Autodesk Inventor part; units mm, degrees
ref_plane "a1_XY" through (0, 12.7, -25.2476) normal (0, 1, 0) x (1, 0, 0)
ref_plane "a1_YZ" through (0, 12.7, -25.2476) normal (1, 0, 0) x (0, 0, -1)
ref_plane "a1_ZX" through (0, 12.7, -25.2476) normal (0, 0, -1) x (0, 1, 0)
sketch "Sketch_1" plane through (0, 0, 0) normal (0, 0, 1) x (1, 0, 0)
  line L0 (0, 0) -> (0, 12.7)
  line L1 (0, 12.7) -> (25.2476, 12.7)
  line L2 (25.2476, 12.7) -> (25.2476, 0)
  line L3 (25.2476, 0) -> (0, 0)
  line L4 (0, 0) -> (0, 12.7)
revolve "Revolution1" add sketch "Sketch_1" angle 360 about axis through (0, 0, 0) along (0, -1, 0)
sketch "Sketch_84" plane through (0, 0, 0) normal (0, 0, 1) x (1, 0, 0)
  line L0 (-16.2306, 5.588) -> (-25.2476, 5.588)
  line L1 (-25.2476, 5.588) -> (-25.2476, 11.0427)
  line L2 (-25.2476, 11.0427) -> (-24.6126, 10.4077)
  line L3 (-24.6126, 10.4077) -> (-16.2306, 10.146)
  line L4 (-16.2306, 10.146) -> (-16.2306, 5.588)
  line L5 (-16.2306, 5.588) -> (-25.2476, 5.588)
revolve "Revolution2" cut sketch "Sketch_84" angle 360 about axis through (-16.2306, 5.588, 0) along (1, 0, 0)
thread "Thread1"
sketch "Sketch_85" plane through (0, 0, 0) normal (0, 0, 1) x (1, 0, 0)
  line L0 (-12.2936, 8.8138) -> (-25.2476, 8.8138)
  line L1 (-25.2476, 8.8138) -> (-25.2476, 10.4013)
  line L2 (-25.2476, 10.4013) -> (-13.2101, 10.4013)
  line L3 (-13.2101, 10.4013) -> (-12.2936, 8.8138)
  line L4 (-12.2936, 8.8138) -> (-25.2476, 8.8138)
revolve "Revolution3" cut sketch "Sketch_85" angle 360 about axis through (-12.2936, 8.8138, 0) along (1, 0, 0)
sketch "Sketch4" plane through (0, 12.7, 0) normal (0, 1, 0) x (1, 0, 0)
  point P0 (-15.1587, -15.1587)
hole "Hole1" at (-15.1587, 12.7, 15.1587) direction (0, -1, 0) diameter 3.9624 depth 12.7 counterbore diameter 5.7404 counterbore depth 3.7592
sketch "Sketch5" plane through (0, 12.7, 0) normal (0, 1, 0) x (1, 0, 0)
  point P0 (15.1587, -15.1587)
hole "Hole2" at (15.1587, 12.7, 15.1587) direction (0, -1, 0) diameter 3.9624 depth 12.7 counterbore diameter 5.7404 counterbore depth 3.7592
sketch "Sketch6" plane through (0, 12.7, 0) normal (0, 1, 0) x (1, 0, 0)
  point P0 (15.1587, 15.1587)
hole "Hole3" at (15.1587, 12.7, -15.1587) direction (0, -1, 0) diameter 3.9624 depth 12.7 counterbore diameter 5.7404 counterbore depth 3.7592
sketch "Sketch7" plane through (0, 12.7, 0) normal (0, 1, 0) x (1, 0, 0)
  point P0 (-15.1587, 15.1587)
hole "Hole4" at (-15.1587, 12.7, -15.1587) direction (0, -1, 0) diameter 3.9624 depth 12.7 counterbore diameter 5.7404 counterbore depth 3.7592
sketch "Sketch8" plane through (0, 0, 0) normal (0, -1, 0) x (1, 0, 0)
  point P0 (0, 0)
hole "Hole5" at (0, 0, 0) direction (0, 1, 0) diameter 28.4988 depth 5.5372
sketch "Sketch9" plane through (0, 12.7, 0) normal (0, 1, 0) x (1, 0, 0)
  point P0 (-18.257, -7.5623)
hole "Hole6" at (-18.257, 12.7, 7.5623) direction (0, -1, 0) diameter 2.6416 depth 12.7 counterbore diameter 3.81 counterbore depth 2.54
pattern_linear "Rectangular Pattern1" count 2 spacing 27.9466 along (0.3827, 0, -0.9239) count 2 spacing 27.9466 along (0.9239, 0, 0.3827) of "Hole6"
ref_plane "a1_XY" through (0, 12.7, -25.2476) normal (0, 1, 0) x (1, 0, 0)
ref_plane "a1_YZ" through (0, 12.7, -25.2476) normal (1, 0, 0) x (0, 0, -1)
ref_plane "a1_ZX" through (0, 12.7, -25.2476) normal (0, 0, -1) x (0, 1, 0)
ref_plane "a2_XY" through (0, 12.7, 25.2476) normal (0, 1, 0) x (1, 0, 0)
ref_plane "a2_YZ" through (0, 12.7, 25.2476) normal (1, 0, 0) x (0, 0, -1)
ref_plane "a2_ZX" through (0, 12.7, 25.2476) normal (0, 0, -1) x (0, 1, 0)
ref_plane "ar3_XY" through (-19.8292, 5.5372, 8.2135) normal (0, 1, 0) x (1, 0, 0)
ref_plane "ar3_YZ" through (-19.8292, 5.5372, 8.2135) normal (1, 0, 0) x (0, 0, -1)
ref_plane "ar3_ZX" through (-19.8292, 5.5372, 8.2135) normal (0, 0, -1) x (0, 1, 0)
ref_plane "ar4_XY" through (8.2135, 5.5372, 19.8292) normal (0, 1, 0) x (1, 0, 0)
ref_plane "ar4_YZ" through (8.2135, 5.5372, 19.8292) normal (1, 0, 0) x (0, 0, -1)
ref_plane "ar4_ZX" through (8.2135, 5.5372, 19.8292) normal (0, 0, -1) x (0, 1, 0)
ref_plane "ar5_XY" through (19.8292, 5.5372, -8.2135) normal (0, 1, 0) x (1, 0, 0)
ref_plane "ar5_YZ" through (19.8292, 5.5372, -8.2135) normal (1, 0, 0) x (0, 0, -1)
ref_plane "ar5_ZX" through (19.8292, 5.5372, -8.2135) normal (0, 0, -1) x (0, 1, 0)
ref_plane "ar6_XY" through (-8.2135, 5.5372, -19.8292) normal (0, 1, 0) x (1, 0, 0)
ref_plane "ar6_YZ" through (-8.2135, 5.5372, -19.8292) normal (1, 0, 0) x (0, 0, -1)
ref_plane "ar6_ZX" through (-8.2135, 5.5372, -19.8292) normal (0, 0, -1) x (0, 1, 0)
ref_plane "b1_XY" through (0, 12.7, 0) normal (0, 1, 0) x (1, 0, 0)
ref_plane "b1_YZ" through (0, 12.7, 0) normal (1, 0, 0) x (0, 0, -1)
ref_plane "b1_ZX" through (0, 12.7, 0) normal (0, 0, -1) x (0, 1, 0)
ref_plane "c11_XY" through (15.1587, 12.7, 15.1587) normal (0, 1, 0) x (1, 0, 0)
ref_plane "c11_YZ" through (15.1587, 12.7, 15.1587) normal (1, 0, 0) x (0, 0, -1)
ref_plane "c11_ZX" through (15.1587, 12.7, 15.1587) normal (0, 0, -1) x (0, 1, 0)
ref_plane "c22_XY" through (-15.1587, 12.7, -15.1587) normal (0, 1, 0) x (1, 0, 0)
ref_plane "c22_YZ" through (-15.1587, 12.7, -15.1587) normal (1, 0, 0) x (0, 0, -1)
ref_plane "c22_ZX" through (-15.1587, 12.7, -15.1587) normal (0, 0, -1) x (0, 1, 0)
ref_plane "d11_XY" through (-16.5596, 12.7, -13.7578) normal (0, 1, 0) x (1, 0, 0)
ref_plane "d11_YZ" through (-16.5596, 12.7, -13.7578) normal (1, 0, 0) x (0, 0, -1)
ref_plane "d11_ZX" through (-16.5596, 12.7, -13.7578) normal (0, 0, -1) x (0, 1, 0)
ref_plane "d22_XY" through (-13.7578, 12.7, -16.5596) normal (0, 1, 0) x (1, 0, 0)
ref_plane "d22_YZ" through (-13.7578, 12.7, -16.5596) normal (1, 0, 0) x (0, 0, -1)
ref_plane "d22_ZX" through (-13.7578, 12.7, -16.5596) normal (0, 0, -1) x (0, 1, 0)
ref_plane "j_XY" through (0, 0, 0) normal (0, 1, 0) x (1, 0, 0)
ref_plane "j_YZ" through (0, 0, 0) normal (1, 0, 0) x (0, 0, -1)
ref_plane "j_ZX" through (0, 0, 0) normal (0, 0, -1) x (0, 1, 0)
ref_plane "k1_XY" through (-25.2476, 5.588, 0) normal (0, 0, 1) x (1, 0, 0)
ref_plane "k1_YZ" through (-25.2476, 5.588, 0) normal (1, 0, 0) x (0, 1, 0)
ref_plane "k1_ZX" through (-25.2476, 5.588, 0) normal (0, 1, 0) x (0, 0, 1)
ref_plane "k2_XY" through (-25.2476, 12.7, 0) normal (0, 0, 1) x (1, 0, 0)
ref_plane "k2_YZ" through (-25.2476, 12.7, 0) normal (1, 0, 0) x (0, 1, 0)
ref_plane "k2_ZX" through (-25.2476, 12.7, 0) normal (0, 1, 0) x (0, 0, 1)
ref_plane "po1_XY" through (19.7612, 0, 0) normal (0, 1, 0) x (1, 0, 0)
ref_plane "po1_YZ" through (19.7612, 0, 0) normal (1, 0, 0) x (0, 0, -1)
ref_plane "po1_ZX" through (19.7612, 0, 0) normal (0, 0, -1) x (0, 1, 0)
ref_plane "po2_XY" through (-8.3514, 0, -17.9097) normal (0, 1, 0) x (1, 0, 0)
ref_plane "po2_YZ" through (-8.3514, 0, -17.9097) normal (1, 0, 0) x (0, 0, -1)
ref_plane "po2_ZX" through (-8.3514, 0, -17.9097) normal (0, 0, -1) x (0, 1, 0)
ref_plane "po3_XY" through (-8.3514, 0, 17.9097) normal (0, 1, 0) x (1, 0, 0)
ref_plane "po3_YZ" through (-8.3514, 0, 17.9097) normal (1, 0, 0) x (0, 0, -1)
ref_plane "po3_ZX" through (-8.3514, 0, 17.9097) normal (0, 0, -1) x (0, 1, 0)
ref_plane "r7_XY" through (-2.413, 12.7, -21.4376) normal (0, 1, 0) x (1, 0, 0)
ref_plane "r7_YZ" through (-2.413, 12.7, -21.4376) normal (1, 0, 0) x (0, 0, -1)
ref_plane "r7_ZX" through (-2.413, 12.7, -21.4376) normal (0, 0, -1) x (0, 1, 0)
ref_plane "r71_XY" through (0, 12.7, 21.4376) normal (0, 1, 0) x (1, 0, 0)
ref_plane "r71_YZ" through (0, 12.7, 21.4376) normal (1, 0, 0) x (0, 0, -1)
ref_plane "r71_ZX" through (0, 12.7, 21.4376) normal (0, 0, -1) x (0, 1, 0)
ref_plane "r72_XY" through (2.413, 12.7, -21.4376) normal (0, 1, 0) x (1, 0, 0)
ref_plane "r72_YZ" through (2.413, 12.7, -21.4376) normal (1, 0, 0) x (0, 0, -1)
ref_plane "r72_ZX" through (2.413, 12.7, -21.4376) normal (0, 0, -1) x (0, 1, 0)
ref_plane "r73_XY" through (0, 12.7, -21.4376) normal (0, 1, 0) x (1, 0, 0)
ref_plane "r73_YZ" through (0, 12.7, -21.4376) normal (1, 0, 0) x (0, 0, -1)
ref_plane "r73_ZX" through (0, 12.7, -21.4376) normal (0, 0, -1) x (0, 1, 0)
ref_plane "rg_XY" through (0, 12.7, 0) normal (0, 1, 0) x (1, 0, 0)
ref_plane "rg_YZ" through (0, 12.7, 0) normal (1, 0, 0) x (0, 0, -1)
ref_plane "rg_ZX" through (0, 12.7, 0) normal (0, 0, -1) x (0, 1, 0)
ref_plane "rh_XY" through (0, 12.7, 0) normal (0, 1, 0) x (1, 0, 0)
ref_plane "rh_YZ" through (0, 12.7, 0) normal (1, 0, 0) x (0, 0, -1)
ref_plane "rh_ZX" through (0, 12.7, 0) normal (0, 0, -1) x (0, 1, 0)
ref_plane "rs_1_XY" through (-15.1587, 15.2908, -15.1587) normal (0, 1, 0) x (1, 0, 0)
ref_plane "rs_1_YZ" through (-15.1587, 15.2908, -15.1587) normal (1, 0, 0) x (0, 0, -1)
ref_plane "rs_1_ZX" through (-15.1587, 15.2908, -15.1587) normal (0, 0, -1) x (0, 1, 0)
ref_plane "rs_2_XY" through (-15.1587, 15.2908, 15.1587) normal (0, 1, 0) x (1, 0, 0)
ref_plane "rs_2_YZ" through (-15.1587, 15.2908, 15.1587) normal (1, 0, 0) x (0, 0, -1)
ref_plane "rs_2_ZX" through (-15.1587, 15.2908, 15.1587) normal (0, 0, -1) x (0, 1, 0)
ref_plane "rs_3_XY" through (15.1587, 15.2908, 15.1587) normal (0, 1, 0) x (1, 0, 0)
ref_plane "rs_3_YZ" through (15.1587, 15.2908, 15.1587) normal (1, 0, 0) x (0, 0, -1)
ref_plane "rs_3_ZX" through (15.1587, 15.2908, 15.1587) normal (0, 0, -1) x (0, 1, 0)
ref_plane "rs_4_XY" through (15.1587, 15.2908, -15.1587) normal (0, 1, 0) x (1, 0, 0)
ref_plane "rs_4_YZ" through (15.1587, 15.2908, -15.1587) normal (1, 0, 0) x (0, 0, -1)
ref_plane "rs_4_ZX" through (15.1587, 15.2908, -15.1587) normal (0, 0, -1) x (0, 1, 0)
ref_plane "sc1_XY" through (19.7612, 8.128, 0) normal (0, 1, 0) x (1, 0, 0)
ref_plane "sc1_YZ" through (19.7612, 8.128, 0) normal (1, 0, 0) x (0, 0, -1)
ref_plane "sc1_ZX" through (19.7612, 8.128, 0) normal (0, 0, -1) x (0, 1, 0)
ref_plane "sc2_XY" through (-8.3514, 8.128, -17.9097) normal (0, 1, 0) x (1, 0, 0)
ref_plane "sc2_YZ" through (-8.3514, 8.128, -17.9097) normal (1, 0, 0) x (0, 0, -1)
ref_plane "sc2_ZX" through (-8.3514, 8.128, -17.9097) normal (0, 0, -1) x (0, 1, 0)
ref_plane "sc3_XY" through (-8.3514, 8.128, 17.9097) normal (0, 1, 0) x (1, 0, 0)
ref_plane "sc3_YZ" through (-8.3514, 8.128, 17.9097) normal (1, 0, 0) x (0, 0, -1)
ref_plane "sc3_ZX" through (-8.3514, 8.128, 17.9097) normal (0, 0, -1) x (0, 1, 0)
ref_plane "to_dummy_XY" through (0, 12.7, 0) normal (0, 1, 0) x (1, 0, 0)
ref_plane "to_dummy_YZ" through (0, 12.7, 0) normal (1, 0, 0) x (0, 0, -1)
ref_plane "to_dummy_ZX" through (0, 12.7, 0) normal (0, 0, -1) x (0, 1, 0)
ref_plane "to_nut_XY" through (0, 16.002, 0) normal (0, 1, 0) x (1, 0, 0)
ref_plane "to_nut_YZ" through (0, 16.002, 0) normal (1, 0, 0) x (0, 0, -1)
ref_plane "to_nut_ZX" through (0, 16.002, 0) normal (0, 0, -1) x (0, 1, 0)
ref_plane "to_rod_XY" through (0, 12.7, 0) normal (0, 1, 0) x (1, 0, 0)
ref_plane "to_rod_YZ" through (0, 12.7, 0) normal (1, 0, 0) x (0, 0, -1)
ref_plane "to_rod_ZX" through (0, 12.7, 0) normal (0, 0, -1) x (0, 1, 0)
ref_plane "to_tube_XY" through (0, 5.5372, 0) normal (0, 1, 0) x (1, 0, 0)
ref_plane "to_tube_YZ" through (0, 5.5372, 0) normal (1, 0, 0) x (0, 0, -1)
ref_plane "to_tube_ZX" through (0, 5.5372, 0) normal (0, 0, -1) x (0, 1, 0)
ref_plane "to_wiper_XY" through (0, 12.7, 0) normal (0, 1, 0) x (1, 0, 0)
ref_plane "to_wiper_YZ" through (0, 12.7, 0) normal (1, 0, 0) x (0, 0, -1)
ref_plane "to_wiper_ZX" through (0, 12.7, 0) normal (0, 0, -1) x (0, 1, 0)
ref_plane "track1_XY" through (-13.0556, 0, 0) normal (0, 1, 0) x (1, 0, 0)
ref_plane "track1_YZ" through (-13.0556, 0, 0) normal (1, 0, 0) x (0, 0, -1)
ref_plane "track1_ZX" through (-13.0556, 0, 0) normal (0, 0, -1) x (0, 1, 0)
ref_plane "track2_XY" through (0, 0, -13.0556) normal (0, 1, 0) x (1, 0, 0)
ref_plane "track2_YZ" through (0, 0, -13.0556) normal (1, 0, 0) x (0, 0, -1)
ref_plane "track2_ZX" through (0, 0, -13.0556) normal (0, 0, -1) x (0, 1, 0)
ref_plane "track3_XY" through (13.0556, 0, 0) normal (0, 1, 0) x (1, 0, 0)
ref_plane "track3_YZ" through (13.0556, 0, 0) normal (1, 0, 0) x (0, 0, -1)
ref_plane "track3_ZX" through (13.0556, 0, 0) normal (0, 0, -1) x (0, 1, 0)
ref_plane "track4_XY" through (0, 0, 13.0556) normal (0, 1, 0) x (1, 0, 0)
ref_plane "track4_YZ" through (0, 0, 13.0556) normal (1, 0, 0) x (0, 0, -1)
ref_plane "track4_ZX" through (0, 0, 13.0556) normal (0, 0, -1) x (0, 1, 0)
properties part number "09-2-0.125-FO1_BM_heads_left-bif"
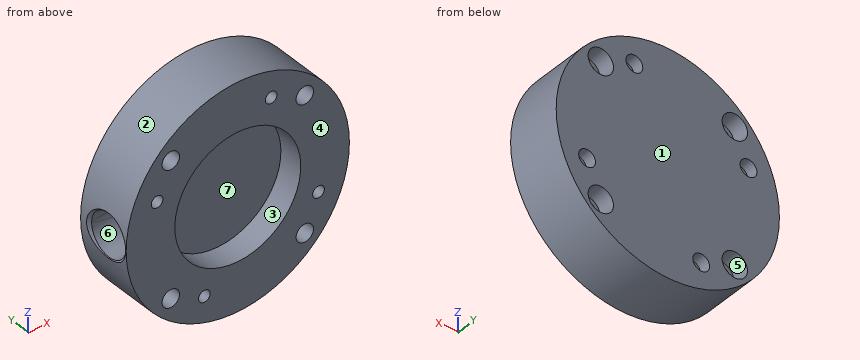
Build history of the part. All positions in model axes, mm. Face numbers are marked on the shaded views. A direction names the side the tool comes from. Round coordinates to 2 decimals unless told otherwise and drop trailing zeros. Order: outer loops, then holes, each group sorted by start corner. A loop starts at its lowest first (then second) coordinate and runs counter-clockwise, first axis right, second up. Notation, with made-up numbers: (84.25, 76) -> (88.25, 76) arc R8 cw to (88.25, 89) -> close; hole circle Ø1 at (50, 37). An arc over 180 degrees is marked (long way). Answer in a Markdown table with one row per item.
1) Band-saw the part on D-D on z = 21. Give the cut face in (x, y).
Values:
| item | result |
|---|---|
| outline | (-14.02, 0) -> (14.02, 0) -> (14.02, 12.7) -> (-14.02, 12.7) -> close |
2) Mould opens along Z. For the marked faces 1, 2 and 3 say: released by +Z, released by -Z, zero draft, split by the parting line, or undercut.
Values:
| item | result |
|---|---|
| face 1 | zero draft |
| face 2 | split by the parting line |
| face 3 | undercut |
3) Band-saw the part on B-B on y = 3.75. Give the number of separate pieces and of enclosed holes in the cut face, and give its area (3 significant figures).
Values:
| item | result |
|---|---|
| separate pieces | 1 |
| enclosed holes | 9 |
| area | 1,220 mm2 |
4) Which spindle directions (+Z, -Z, +X, -X, +Y, -Y) get a long thin tool onto all of the face, cutting with end or side? Do the marked faces 4, 5, 6 and 7. Say none if no direction does.
Values:
| item | result |
|---|---|
| face 4 | +Z, -Z, +X, -X, -Y |
| face 5 | +Y |
| face 6 | -X |
| face 7 | -Y |
5) Pin check, flat tips, straight feed: P1, Ø1, axis at y = 10, z = 17, coming from the -X side; P2, Ø3, axis at x = -18, z = 8, coming from the +Y side; P3, Ø2, axis at x = 17, y = 11, coming from the +Z side; P4, Ø1.5, axis at y = 9, z = 11.5, coming from the +X side. Stop position of each tip, or through.
Values:
| item | result |
|---|---|
| P1 | x = -19.11 |
| P2 | y = 12.7 |
| P3 | z = 19.53 |
| P4 | x = 22.84 |
6) Band-saw the part on A-A on x = 0. Give the cut face in (y, z).
Values:
| item | result |
|---|---|
| outline | (0, -25.25) -> (12.7, -25.25) -> (12.7, 25.25) -> (0, 25.25) -> (0, 14.25) -> (5.54, 14.25) -> (5.54, -14.25) -> (0, -14.25) -> close |
7) Wall check: L1, parallel to Y at x = -16.5, z = 0; L2, parallel to Z at x = -12, y = 3.75; L3, parallel to X at y = 5, z = 6. Give the ranges that are in metal, low to high.
Values:
| item | result |
|---|---|
| L1 | 0 to 1.02, 10.4 to 12.7 |
| L2 | -22.21 to -7.68, 7.68 to 22.21 |
| L3 | -24.52 to -12.92, 12.92 to 24.52 |
